Source: CAD feature listing. Evaluate the final solid. Frame: model axes, mm. A direction names the side the tool comes from. Coordinates: 2 decimals unless noted, no trailing zeros. Loops run counter-clockwise (first coordinate to the right, second up) from the corner with the lowest first, then second, coordinate; pieces in that order, holes last. Notation, with made-up numbers: (0, 47) -> (18, 47) arc R18 cw to (18, 51) -> close; hole circle Ø1 at (5, 57). An arc over 180 degrees is marked (long way). Answer as CSV lines item,"result".
from build123d import *

# Parameters (mm, degrees)
F0_R     = 20.25
F0_R_2   = 7.75
F1_DEPTH = 2
F2_R     = 22.25
F2_R_2   = 20.25
F3_DEPTH = 5
F4_SIZE  = 0.5
F5_SIZE  = 1


with BuildPart() as f1:
    # F0 (on Top) → F1 (new body)
    with BuildSketch(Plane.XY):
        Circle(F0_R)
        Circle(F0_R_2, mode=Mode.SUBTRACT)
    extrude(amount=F1_DEPTH)

    # F2 (on face) → F3 (join)
    with BuildSketch(Plane.XY.offset(2)):
        Circle(F2_R)
        Circle(F2_R_2, mode=Mode.SUBTRACT)
    extrude(amount=-F3_DEPTH)

    # F4
    f4_edges = [f1.edges().sort_by_distance(p)[0] for p in [
        (-7.75, 0, 0),
    ]]
    chamfer(f4_edges, length=F4_SIZE)

    # F5
    f5_edges = [f1.edges().sort_by_distance(p)[0] for p in [
        (-22.25, 0, 2),
    ]]
    chamfer(f5_edges, length=F5_SIZE)


solid = f1.part
(1) Pin query (flat end, axial travel): pin 1 Ø14 at (x, y) = (0, 0) entering from -Z; pin 2 Ø4 at (x, y) = (-16.5, 8) entering from -Z; pin 3 Ø2 at (x, z) = (-6, 0) entering from -Y; pin 4 Ø1.5 at (x, z) = (-10.5, 0.5) entering from -Y. Return the tip coordinate at first contact, or that it passes through.
Computed values:
pin 1,"through"
pin 2,"z = -3"
pin 3,"y = -21.68"
pin 4,"y = -20"
(2) Cut plane C-C (z = -2.2). Return the cut outline in (x, y), then the cut area to 3 significant figures.
Computed values:
outline,"circle Ø44.5 at (0, 0); hole circle Ø40.5 at (0, 0)"
area,"267 mm^2"
(3) Access query for faces 1 (the cylindrical face through (-1.009, 7.684, 1.24)), 2 (the flat face through (0, -9, 0)). Directions: +Z, -Z, +X, -X, +Y, -Y. A direction counts if a zero-diameter tool reaches every point of the face in a straight line with its end or side. Return the directions, or none.
Computed values:
face 1,"+Z, -Z"
face 2,"-Z"
(4) Material intervals for L1, parallel to Y at x = 0, z = -1.65; L2, parallel to Y at x = 0, z = 1; L3, parallel to X at y = -10.5, z = -1.55, sorted ascending. Write a range as [from, to].
Computed values:
L1,"[-22.25, -20.25], [20.25, 22.25]"
L2,"[-22.25, -7.75], [7.75, 22.25]"
L3,"[-19.62, -17.32], [17.32, 19.62]"
(5) Cut plane A-A (x = 0). Return the cut outline in (y, z).
Computed values:
outline,"(-22.25, -3) -> (-20.25, -3) -> (-20.25, 0) -> (-8.25, 0) -> (-7.75, 0.5) -> (-7.75, 2) -> (-21.25, 2) -> (-22.25, 1) -> close; (7.75, 0.5) -> (8.25, 0) -> (20.25, 0) -> (20.25, -3) -> (22.25, -3) -> (22.25, 1) -> (21.25, 2) -> (7.75, 2) -> close"
